Could you check a few things on this model? Use its own coordinates, in mm. Give positions to 0.01 mm unless a question says otherwise; leave off trailing zeros. Order: outer loops, then holes, each group sorted by start corner. A loop starts at its lowest first (then second) coordinate and runs counter-clockwise, first axis right, second up. Notation, with made-up numbers: (43.25, 60) -> (96.25, 60) arc R23 cw to (96.25, 69) -> close; hole circle Ø9 at (61.25, -16). An arc over 180 degrees is marked (long way). Answer as CSV lines item,"result". Start each with the question number.
(1) I want a section at C-C (y = 7.75). Please give me the cut outline in (x, z) (3 decimals), plus the area to 3 significant figures.
(2) Will these pins go through, and if not, where does the flat tip stop? pin 1 Ø1.6 at (y, z) = (15.5, 1) entering from +X; pin 2 Ø1.6 at (x, z) = (2.5, 1.5) entering from -Y; pin 3 Ø1 at (x, z) = (2, 1.5) entering from +Y.
(3) I want a section at B-B (z = 2.5). Please give me the cut outline in (x, y) (1 decimal), plus the area to 3 significant figures.
(4) I want a section at D-D (y = 2.5). Please give me the cut outline in (x, z) (3 decimals).
(5) I want a section at A-A (x = -92). Please give me the cut outline in (y, z) (3 decimals).
(6) I need wall thicknesses on L1, parallel to Y at x = -17, z = 2.7; L2, parallel to X at y = 3, z = 2.1; L3, parallel to X at y = 6.25, z = 2.45 (3 decimals). Which ranges of each line are inside material? Lowest first, please.
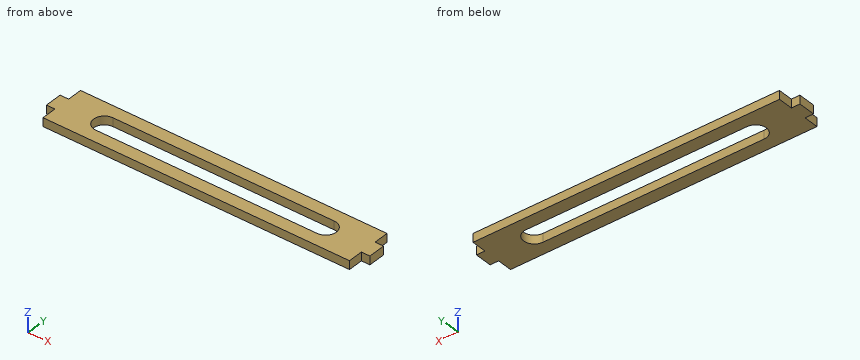
```python
from build123d import *

# Parameters (mm, degrees)
BOSS_EXTRUDE1_DEPTH = 3.175
CUT_EXTRUDE2_DEPTH  = 4.175


with BuildPart() as part:
    # Sketch1 → Boss-Extrude1 (new body)
    with BuildSketch(Plane.XY):
        Polygon((0, 0), (-114.3, 0), (-114.3, 5.555107), (-117.475, 5.555107), (-117.475, 11.905107), (-114.3, 11.905107), (-114.3, 17.460214), (0, 17.460214), (0, 11.905107), (3.175, 11.905107), (3.175, 5.555107), (0, 5.555107), align=None)
    extrude(amount=BOSS_EXTRUDE1_DEPTH)

    # Sketch3 → Cut-Extrude2 (cut, through all)
    with BuildSketch(Plane.XY.offset(3.175)):
        with BuildLine():
            Line((-15.875, 4.761357), (-98.425, 4.761357))
            ThreePointArc((-98.425, 4.761357), (-102.39375, 8.730107), (-98.425, 12.698857))
            Line((-98.425, 12.698857), (-15.875, 12.698857))
            ThreePointArc((-15.875, 12.698857), (-11.90625, 8.730107), (-15.875, 4.761357))
        make_face()
    extrude(amount=-CUT_EXTRUDE2_DEPTH, mode=Mode.SUBTRACT)


solid = part.part
```
Final values:
1,outline,"(-117.475, 0) -> (-102.271, 0) -> (-102.271, 3.175) -> (-117.475, 3.175) -> close; (-12.029, 0) -> (3.175, 0) -> (3.175, 3.175) -> (-12.029, 3.175) -> close"
1,area,"96.5 mm²"
2,pin 1,"x = 0"
2,pin 2,"y = 5.56"
2,pin 3,"y = 11.91"
3,outline,"(-117.5, 5.6) -> (-114.3, 5.6) -> (-114.3, 0) -> (0, 0) -> (0, 5.6) -> (3.2, 5.6) -> (3.2, 11.9) -> (0, 11.9) -> (0, 17.5) -> (-114.3, 17.5) -> (-114.3, 11.9) -> (-117.5, 11.9) -> close; hole (-98.4, 4.8) -> (-15.9, 4.8) arc R4 ccw to (-15.9, 12.7) -> (-98.4, 12.7) arc R4 ccw to start"
3,area,"1,330 mm²"
4,outline,"(-114.3, 0) -> (0, 0) -> (0, 3.175) -> (-114.3, 3.175) -> close"
5,outline,"(0, 0) -> (4.761, 0) -> (4.761, 3.175) -> (0, 3.175) -> close; (12.699, 0) -> (17.46, 0) -> (17.46, 3.175) -> (12.699, 3.175) -> close"
6,L1,"0 to 4.76, 12.7 to 17.46"
6,L2,"-114.3 to 0"
6,L3,"-117.475 to -101.523, -12.777 to 3.175"
